from build123d import *

# Parameters (mm, degrees)
BOSS_EXTRUDE1_DEPTH = 120
FILLET1_R           = 4


with BuildPart() as part:
    # Sketch1 → Boss-Extrude1 (new body)
    with BuildSketch(Plane(origin=(0, 0, 0), x_dir=(1, 0, 0), z_dir=(0, 1, 0))):
        Polygon((145, 0), (0, 0), (0, 145), (-3, 145), (-3, -3), (145, -3), align=None)
    extrude(amount=BOSS_EXTRUDE1_DEPTH)

    # Fillet1
    fillet1_edges = [part.edges().sort_by_distance(p)[0] for p in [
        (-3, 60, 3),
    ]]
    fillet(fillet1_edges, radius=FILLET1_R)


solid = part.part
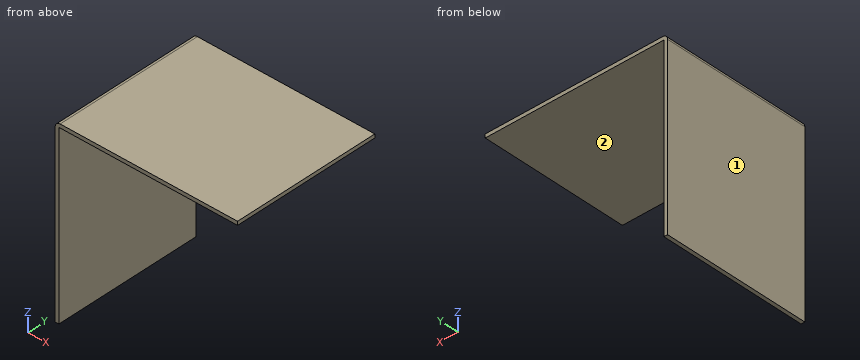
The model under review builds one solid part; all positions refer to its coordinate system, in mm. Face numbers are marked on the shaded views. A direction names the side the tool comes from. Coordinates: 2 decimals unless noted, no trailing zeros. Write each loop counter-clockwise with the first axis right and the second up, starting at its lowest first coordinate (ties: lowest second). Pieces come first, ordered by that corner, then holes. Notation, with made-up numbers: (5.5, 65) - (33.5, 65) arc R34 cw to (33.5, 96) - close; hole circle Ø10 at (-35, 26.25). An arc over 180 degrees is marked (long way). Answer as a JSON object with one key per item and string values. Group by question number.
1. Add section A-A (y = 52.5). Give the boundary of the cut face in (x, z), plus the area to 3 significant figures.
2. Clearance check with flat-ended pins moving along their axes: pin 1 Ø10 at (y, z) = (105, -76) entering from +X; pin 2 Ø1 at (x, y) = (70, 46.5) entering from -Z. State where each tip first meets the part, or that it passes through.
3. Machinability: for the marked faces 1 and 2, which of the approach directions +Z, -Z, +X, -X, +Y, -Y give a long, thin tool a straight path to every point of the face, cutting with its end or side? Answer none if there is none.
4. Add section B-B (x = 54.5). Give the boundary of the cut face in (y, z), plus the area to 3 significant figures.
5. To check wall thickness, follow probe 1 along Z at (x, y) = (72.5, 42); probe 2 along X at (y, z) = (32.5, -73). State the ranges of each line that lie inside material, in increasing order.
6. Add section C-C (z = -100). Give the boundary of the cut face in (x, y), plus the area to 3 significant figures.
Findings:
{
 "1": {"outline": "(-3, -145) - (0, -145) - (0, 0) - (145, 0) - (145, 3) - (1, 3) arc R4 ccw to (-3, -1) - close", "area": "876 mm²"},
 "2": {"pin 1": "x = 0", "pin 2": "z = 0"},
 "3": {"face 1": "+Z, -Z, -X, +Y, -Y", "face 2": "-Z, +X, +Y, -Y"},
 "4": {"outline": "(0, 0) - (120, 0) - (120, 3) - (0, 3) - close", "area": "360 mm²"},
 "5": {"probe 1": "0 to 3", "probe 2": "-3 to 0"},
 "6": {"outline": "(-3, 0) - (0, 0) - (0, 120) - (-3, 120) - close", "area": "360 mm²"}
}
